Model file for the job. Use its own axes, mm. Face numbers are marked on the shaded views. A direction names the side the tool comes from. Give positions to 0.01 mm unless a question says otherwise; leave off trailing zeros. Order: outer loops, then holes, each group sorted by start corner. A loop starts at its lowest first (then second) coordinate and runs counter-clockwise, first axis right, second up. Notation, with made-up numbers: M 50,61 L 63,61 A9 ccw 63,77 Z; hole C 8,89.25 d5. An arc over 180 degrees is marked long. Return JSON: item names as keys, results as strings. Group by question number.
1. Slice it at B-B on y = 19. List the corners of the cut face in (x, z).
2. Slice it at C-C on x = 27.5. List the corners of the cut face in (y, z), then the cut area to 3 significant figures.
3. Wall check: probe 1 along Y at (x, z) = (41.5, 10); probe 2 along Z at (x, y) = (7, 33.5). Give the ranges that are in metal, low to high. Write a range as [from, to].
4. 3-axis set-ups, long thin cutter, end or side, ignore diameter. For the marked faces 1, 2, 3, 4 and 5: which of +Z, -Z, +X, -X, +Y, -Y reach the whole face in a straight line?
5. Slice it at A-A on z = 9. List the corners of the cut face in (x, y), then the cut area to 3 significant figures.
6. Slice it at D-D on z = 24. List the corners of the cut face in (x, y), then the cut area to 3 significant figures.
7. Pin check, flat tips, straight feed: pin 1 (2.5 mm diameter, centred on x = 32, y = 2, fed in from +Z); pin 2 (2.5 mm diameter, centred on x = 10, z = 38, fed in from +Y); pin 3 (0.9 mm diameter, centred on x = 39, y = 6, fed in from +Z). Stop position of each tip, or through.
8. Two-plate mould, pull along Y, no slides. Class the marked faces 6, 7 and 8: released by +Y, released by -Y, zero draft, split by the parting line, or undercut.
from build123d import *

# Parameters (mm, degrees)
PAD_DEPTH     = 13
SKETCH001_W   = 13
SKETCH001_H   = 13.105825
PAD001_DEPTH  = 50
SKETCH002_W   = 70.608528
SKETCH002_H   = 3
SKETCH002_W_2 = 3
SKETCH002_H_2 = 60
POCKET_DEPTH  = 45
PAD003_DEPTH  = 5
PAD004_DEPTH  = 10
FILLET002_R   = 1
FILLET_R      = 1


with BuildPart() as part:
    # Sketch → Pad (new body)
    with BuildSketch(Plane.XY):
        Polygon((0, 0), (50, 0), (50, 13), (13, 13), (13, 50), (0, 50), align=None)
    extrude(amount=PAD_DEPTH)

    # Sketch001 → Pad001 (join)
    with BuildSketch(Plane.XY):
        with Locations((6.5, 6.5529125)):
            Rectangle(SKETCH001_W, SKETCH001_H)
    extrude(amount=PAD001_DEPTH)

    # Sketch002 (on Face7 of Pad001) → Pocket (cut)
    with BuildSketch(Plane.XY.offset(50)):
        with Locations((45.304264, 6.5)):
            Rectangle(SKETCH002_W, SKETCH002_H)
        with Locations((6.5, 40)):
            Rectangle(SKETCH002_W_2, SKETCH002_H_2)
    extrude(amount=-POCKET_DEPTH, mode=Mode.SUBTRACT)

    # Sketch004 → Pad003 (join)
    with BuildSketch(Plane.XZ):
        with BuildLine():
            Line((8, 8), (23, 8))
            Line((23, 8), (23, 21))
            ThreePointArc((23, 21), (22.4142135624, 22.4142135624), (21, 23))
            Line((21, 23), (8, 23))
            Line((8, 23), (8, 8))
        make_face()
    extrude(amount=-PAD003_DEPTH)

    # Sketch005 → Pad004 (join)
    with BuildSketch(Plane.XZ):
        with BuildLine():
            Line((21, 23), (15, 23))
            ThreePointArc((15, 23), (13.5857864376, 22.4142135623), (13, 20.9999999999))
            Line((13, 20.9999999999), (13, 15))
            ThreePointArc((13, 15), (13.5857864376, 13.5857864376), (15, 13))
            Line((15, 13), (21, 13))
            ThreePointArc((21, 13), (22.4142135624, 13.5857864376), (23, 15))
            Line((23, 15), (23, 20.9999999999))
            ThreePointArc((23, 20.9999999999), (22.4142135624, 22.4142135623), (21, 23))
        make_face()
    extrude(amount=PAD004_DEPTH)

    # Fillet002
    fillet002_edges = [part.edges().sort_by_distance(p)[0] for p in [
        (18, -10, 23),
        (13.585786, -10, 22.414214),
        (13, -10, 18),
        (13.585786, -10, 13.585786),
        (18, -10, 13),
        (22.414214, -10, 13.585786),
        (23, -10, 18),
        (22.414214, -10, 22.414214),
    ]]
    fillet(fillet002_edges, radius=FILLET002_R)

    # Fillet
    fillet_edges = [part.edges().sort_by_distance(p)[0] for p in [
        (0, 25, 0),
        (6.5, 50, 0),
        (13, 31.5, 0),
        (31.5, 13, 0),
        (50, 6.5, 0),
        (25, 0, 0),
        (0, 0, 25),
        (0, 6.552912, 50),
        (0, 13.105825, 31.5),
        (0, 31.552912, 13),
        (0, 50, 6.5),
    ]]
    fillet(fillet_edges, radius=FILLET_R)


solid = part.part
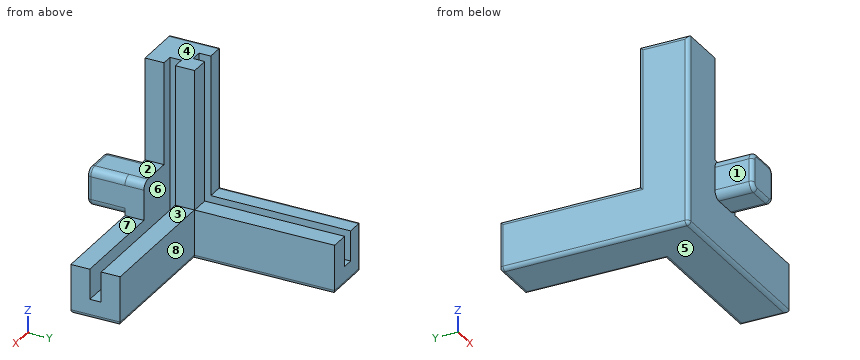
Result:
{
 "1": {"outline": "M 0,1 A1 ccw 1,0 L 12,0 A1 ccw 13,1 L 13,13 L 8,13 L 8,5 L 5,5 L 5,13 L 1,13 A1 ccw 0,12 Z"},
 "2": {"outline": "M 0,1 A1 ccw 1,0 L 12,0 A1 ccw 13,1 L 13,13 L 8,13 L 8,5 L 5,5 L 5,13 L 0,13 Z", "area": "145 mm2"},
 "3": {"probe 1": "y = [0, 5], [8, 13]", "probe 2": "z = [0, 5]"},
 "4": {"face 1": "+Z, -Z, -X, -Y", "face 2": "+Z, +X, +Y, -Y", "face 3": "+Z, +X, +Y", "face 4": "+Z, +X, -X, +Y, -Y", "face 5": "-Z, +X, -X, +Y, -Y"},
 "5": {"outline": "M 0,1 A1 ccw 1,0 L 50,0 L 50,5 L 10,5 L 10,8 L 50,8 L 50,13 L 13,13 L 13,50 L 8,50 L 8,10 L 5,10 L 5,50 L 1,50 A1 ccw 0,49 Z", "area": "891 mm2"},
 "6": {"outline": "M 0,1 A1 ccw 1,0 L 13,0 L 13,5 L 10,5 L 10,8 L 13,8 L 13,13.11 L 8,13.11 L 8,10 L 5,10 L 5,13.11 L 1,13.11 A1 ccw 0,12.11 Z", "area": "152 mm2"},
 "7": {"pin 1": "stops at z = 13", "pin 2": "stops at y = 13.11", "pin 3": "stops at z = 5"},
 "8": {"face 6": "undercut", "face 7": "zero draft", "face 8": "released by +Y"}
}
